Check sheet for the modelled part. Datum: model origin and axes. Units: mm. Coordinates: 2 decimals unless noted, no trailing zeros. Loops run counter-clockwise (first coordinate to the right, second up) from the corner with the lowest first, then second, coordinate; pieces in that order, holes last.
from build123d import *

# Parameters (mm, degrees)
SKETCH2_R           = 2.5
BOSS_EXTRUDE2_DEPTH = 2


with BuildPart() as part:
    # Sketch2 → Boss-Extrude2 (new body)
    with BuildSketch(Plane(origin=(0, 0, 0), x_dir=(1, 0, 0), z_dir=(0, 1, 0))):
        with BuildLine():
            Line((14.393173744, 58.640634372), (-56.574951574, 12.641394771))
            ThreePointArc((-56.574951574, 12.641394771), (-61.135882078, 4.249939413), (-56.574951574, -4.141515944))
            Line((-56.574951574, -4.141515944), (14.393173744, -50.140755545))
            Line((14.393173744, -50.140755545), (14.393173744, 58.640634372))
        make_face()
        with Locations((-51.135882078, 4.249939413)):
            Circle(SKETCH2_R, mode=Mode.SUBTRACT)
        with Locations((-17.570060648, 26.006217397)):
            Circle(SKETCH2_R, mode=Mode.SUBTRACT)
        with Locations((-0.787149932, 36.884356389)):
            Circle(SKETCH2_R, mode=Mode.SUBTRACT)
        with Locations((-17.570060648, -17.50633857)):
            Circle(SKETCH2_R, mode=Mode.SUBTRACT)
        with Locations((-0.787149932, -28.384477562)):
            Circle(SKETCH2_R, mode=Mode.SUBTRACT)
    extrude(amount=BOSS_EXTRUDE2_DEPTH)


solid = part.part
(1) Draft check along X on faces 1 (the face through (-21.59, 0.99, 26.82)), 2 (the face through (-19.41, 0.99, -27.7)), 3 (the face through (14.393, 1, -3)). Enter one of: pulls with the +X half, pulls with the -X half, needs draft (parallel to the pull), parting line crosses it, or undercut.
(2) Section check B-B, the plane x = 0.5. Enter the section's corners in (y, z), plus the area to 3 significant figures.
(3) Scan lines: line 1 along Z through (x, y) = (0, 0.15); line 2 along Z through (x, y) = (-16.5, 0.8); line 3 along X through (y, z) = (0.5, -25). Record each from-to range of solid material in increasing order.
(4) Section check C-C, the plane y = 0.5. Enter the section's corners in (x, z).
(5) Section check A-A, the plane z = -38. Enter the section's corners in (x, y), plus the area to 3 significant figures.
(6) Section check D-D, the plane z = -22. Enter the section's corners in (x, y), plus the area to 3 significant figures.
Determined:
1. face 1: pulls with the -X half
1. face 2: undercut
1. face 3: pulls with the +X half
2. outline: (0, -49.64) - (2, -49.64) - (2, -39.03) - (0, -39.03) - close; (0, -34.74) - (2, -34.74) - (2, 26.24) - (0, 26.24) - close; (0, 30.53) - (2, 30.53) - (2, 41.14) - (0, 41.14) - close
2. area: 164 mm2
3. line 1: z = -49.31 to -39.26, -34.51 to 26.01, 30.76 to 40.81
3. line 2: z = -38.62 to -28.27, -23.75 to 15.25, 19.77 to 30.12
3. line 3: x = -37.51 to -19.86, -15.28 to 14.39
4. outline: (-56.57, -12.64) - (14.39, -58.64) - (14.39, 50.14) - (-56.57, 4.14) arc R10 ccw to start; hole circle Ø5 at (-51.14, -4.25); hole circle Ø5 at (-17.57, -26.01); hole circle Ø5 at (-17.57, 17.51); hole circle Ø5 at (-0.79, -36.88); hole circle Ø5 at (-0.79, 28.38)
5. outline: (-17.45, 0) - (-3.02, 0) - (-3.02, 2) - (-17.45, 2) - close; (1.45, 0) - (14.39, 0) - (14.39, 2) - (1.45, 2) - close
5. area: 54.7 mm2
6. outline: (-42.14, 0) - (14.39, 0) - (14.39, 2) - (-42.14, 2) - close
6. area: 113 mm2
